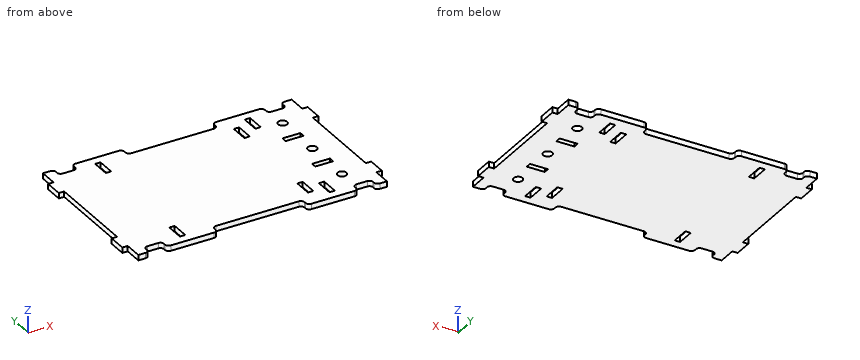
Autodesk Inventor part; units mm, degrees
ref_plane "YZ Plane" through (0, 0, 0) normal (1, 0, 0) x (0, 1, 0)
ref_plane "XZ Plane" through (0, 0, 0) normal (0, 1, 0) x (-1, 0, 0)
ref_plane "XY Plane" through (0, 0, 0) normal (0, 0, 1) x (1, 0, 0)
sketch "Sketch1" plane through (0, 0, 0) normal (0, 0, 1) x (1, 0, 0)
  line L0 (138, 80) -> (141, 80)
  line L1 (141, 80) -> (141, 70)
  line L2 (141, 70) -> (138, 70)
  line L3 (138, 10) -> (141, 10)
  line L4 (141, 10) -> (141, 20)
  line L5 (141, 20) -> (138, 20)
  line L6 (138, 80) -> (138, 90)
  line L7 (138, 20) -> (138, 70)
  line L8 (0, 80) -> (-3, 80)
  line L9 (-3, 80) -> (-3, 70)
  line L10 (-3, 70) -> (0, 70)
  line L11 (0, 20) -> (-3, 20)
  line L12 (-3, 20) -> (-3, 10)
  line L13 (-3, 10) -> (0, 10)
  line L14 (0, 90) -> (0, 80)
  line L15 (0, 70) -> (0, 20)
  line L16 (0, 10) -> (0, 0)
  line L17 (26, 85) -> (29, 85)
  line L18 (29, 85) -> (29, 75)
  line L19 (29, 75) -> (26, 75)
  line L20 (26, 75) -> (26, 85)
  line L21 (26, 15) -> (29, 15)
  line L22 (29, 15) -> (29, 5)
  line L23 (29, 5) -> (26, 5)
  line L24 (26, 5) -> (26, 15)
  line L25 (109, 85) -> (112, 85)
  line L26 (112, 85) -> (112, 75)
  line L27 (112, 75) -> (109, 75)
  line L28 (109, 75) -> (109, 85)
  line L29 (109, 15) -> (112, 15)
  line L30 (112, 15) -> (112, 5)
  line L31 (112, 5) -> (109, 5)
  line L32 (109, 5) -> (109, 15)
  line L33 (16, 88) -> (16, 87)
  line L34 (14, 85) -> (8, 85)
  line L35 (6, 87) -> (6, 88)
  line L36 (94, 88) -> (94, 87)
  line L37 (92, 85) -> (46, 85)
  line L38 (44, 87) -> (44, 88)
  line L39 (132, 88) -> (132, 87)
  line L40 (130, 85) -> (124, 85)
  line L41 (122, 87) -> (122, 88)
  line L42 (138, 90) -> (134, 90)
  line L43 (0, 90) -> (4, 90)
  line L44 (18, 90) -> (42, 90)
  line L45 (96, 90) -> (120, 90)
  line L46 (16, 2) -> (16, 3)
  line L47 (14, 5) -> (8, 5)
  line L48 (6, 3) -> (6, 2)
  line L49 (94, 2) -> (94, 3)
  line L50 (92, 5) -> (46, 5)
  line L51 (44, 3) -> (44, 2)
  line L52 (132, 2) -> (132, 3)
  line L53 (130, 5) -> (124, 5)
  line L54 (122, 3) -> (122, 2)
  line L55 (96, 0) -> (120, 0)
  line L56 (0, 0) -> (4, 0)
  line L57 (18, 0) -> (42, 0)
  arc A0 (4, 0) -> (6, 2) centre (4, 2) ccw
  arc A1 (8, 5) -> (6, 3) centre (8, 3) ccw
  arc A2 (16, 3) -> (14, 5) centre (14, 3) ccw
  arc A3 (16, 2) -> (18, 0) centre (18, 2) ccw
  arc A4 (42, 0) -> (44, 2) centre (42, 2) ccw
  arc A5 (46, 5) -> (44, 3) centre (46, 3) ccw
  arc A6 (94, 3) -> (92, 5) centre (92, 3) ccw
  arc A7 (94, 2) -> (96, 0) centre (96, 2) ccw
  arc A8 (120, 0) -> (122, 2) centre (120, 2) ccw
  arc A9 (124, 5) -> (122, 3) centre (124, 3) ccw
  arc A10 (132, 3) -> (130, 5) centre (130, 3) ccw
  arc A11 (132, 2) -> (134, 0) centre (134, 2) ccw
  arc A12 (6, 88) -> (4, 90) centre (4, 88) ccw
  arc A13 (6, 87) -> (8, 85) centre (8, 87) ccw
  arc A14 (14, 85) -> (16, 87) centre (14, 87) ccw
  arc A15 (18, 90) -> (16, 88) centre (18, 88) ccw
  arc A16 (44, 88) -> (42, 90) centre (42, 88) ccw
  arc A17 (44, 87) -> (46, 85) centre (46, 87) ccw
  arc A18 (92, 85) -> (94, 87) centre (92, 87) ccw
  arc A19 (96, 90) -> (94, 88) centre (96, 88) ccw
  arc A20 (122, 88) -> (120, 90) centre (120, 88) ccw
  arc A21 (122, 87) -> (124, 85) centre (124, 87) ccw
  arc A22 (130, 85) -> (132, 87) centre (130, 87) ccw
  arc A23 (134, 90) -> (132, 88) centre (134, 88) ccw
  line L58 (138, 10) -> (138, 0)
  line L59 (138, 0) -> (134, 0)
  line L60 (103, 10) -> (100, 10)
  line L61 (100, 10) -> (100, 20)
  line L62 (100, 20) -> (103, 20)
  line L63 (103, 20) -> (103, 10)
  line L64 (103, 80) -> (100, 80)
  line L65 (100, 80) -> (100, 70)
  line L66 (100, 70) -> (103, 70)
  line L67 (103, 70) -> (103, 80)
  line L68 (115.5, 60.5) -> (125.5, 60.5)
  line L69 (125.5, 60.5) -> (125.5, 57.5)
  line L70 (125.5, 57.5) -> (115.5, 57.5)
  line L71 (115.5, 57.5) -> (115.5, 60.5)
  line L72 (115.5, 32.5) -> (125.5, 32.5)
  line L73 (125.5, 32.5) -> (125.5, 29.5)
  line L74 (125.5, 29.5) -> (115.5, 29.5)
  line L75 (115.5, 29.5) -> (115.5, 32.5)
  circle A24 centre (123, 45) radius 2.5
  circle A25 centre (123, 73) radius 2.5
  circle A26 centre (123, 17) radius 2.5
  point P0 (16, 85)
  point P1 (6, 85)
  point P2 (94, 85)
  point P3 (44, 85)
  point P4 (132, 85)
  point P5 (122, 85)
  point P6 (16, 5)
  point P7 (6, 5)
  point P8 (94, 5)
  point P9 (44, 5)
  point P10 (132, 5)
  point P11 (122, 5)
  dimension "d1" = 90
  dimension "d3" = 10
  dimension "d4" = 50
  dimension "d5" = 10
  dimension "d10" = 3
  dimension "d11" = 3
  dimension "d13" = 3
  dimension "d14" = 3
  dimension "d16" = 10
  dimension "d17" = 10
  dimension "d20" = 138
  dimension "d21" = 50
  dimension "d22" = 3
  dimension "d23" = 3
  dimension "d24" = 3
  dimension "d27" = 26
  dimension "d28" = 3
  dimension "d30" = 3
  dimension "d31" = 26
  dimension "d33" = 10
  dimension "d34" = 10
  dimension "d35" = 26
  dimension "d36" = 3
  dimension "d38" = 10
  dimension "d39" = 3
  dimension "d40" = 10
  dimension "d45" = 10
  dimension "d46" = 50
  dimension "d47" = 10
  dimension "d48" = 6
  dimension "d49" = 6
  dimension "d54" = 10
  dimension "d55" = 50
  dimension "d56" = 10
  dimension "d57" = 2
  dimension "d58" = 26
  dimension "d59" = 6
  dimension "d60" = 6
  dimension "d62" = 28
  dimension "d63" = 3
  dimension "d64" = 28
  dimension "d65" = 28
  dimension "d66" = 28
  dimension "d67" = 5
  dimension "d68" = 5
  dimension "d69" = 5
  dimension "d70" = 5
  dimension "d71" = 5
  dimension "d72" = 5
  dimension "d73" = 5
  dimension "d74" = 5
  dimension "d75" = 5
  dimension "d76" = 5
  dimension "d77" = 5
  dimension "d78" = 5
  dimension "d79" = 3
  dimension "d80" = 10
  dimension "d81" = 35
  dimension "d82" = 10
  dimension "d83" = 3
  dimension "d84" = 10
  dimension "d85" = 10
  dimension "d86" = 35
  dimension "d89" = 10
extrude "Extrusion5" add sketch "Sketch1" along normal blind 3
properties part number "OpenROV 2.3 Dev EChassis Main Plate"
Can you work these out from the model? Positions are in its coordinate system, mm. Coordinates: 2 decimals unless noted, no trailing zeros. Loops run counter-clockwise (first coordinate to the right, second up) from the corner with the lowest first, then second, coordinate; pieces in that order, holes last.
Item 1: I'm going to push flat-ended pins straight in: pin 1 (0.9 mm diameter, centred on x = -1, z = 2, fed in from +Y); pin 2 (1.5 mm diameter, centred on y = 83.5, z = 2, fed in from +X); pin 3 (1.5 mm diameter, centred on x = 139, z = 1.5, fed in from -Y); pin 4 (4.5 mm diameter, centred on x = 123, y = 17, fed in from +Z). Where does each tip first touch, or does it pass through?
Answers below:
pin 1: stops at y = 80
pin 2: stops at x = 138
pin 3: stops at y = 10
pin 4: passes through
Item 2: Suppose I cut it at B-B (x = 27.5). Please give me the cut outline in (y, z), then the cut area to 3 significant figures.
Answers below:
outline: (0, 0) - (5, 0) - (5, 3) - (0, 3) - close; (15, 0) - (75, 0) - (75, 3) - (15, 3) - close; (85, 0) - (90, 0) - (90, 3) - (85, 3) - close
area: 210 mm2
Item 3: Suppose I cut it at D-D (x = 65.5). Please give me the cut outline in (y, z), then the cut area to 3 significant figures.
Answers below:
outline: (5, 0) - (85, 0) - (85, 3) - (5, 3) - close
area: 240 mm2
Item 4: Please list where these lines run through material, in increasing order: L1, parallel to X at y = 13, z = 1.75; L2, parallel to Y at x = 123, z = 1.05; L3, parallel to X at y = 50, z = 0.5.
Answers below:
L1: x = -3 to 26, 29 to 100, 103 to 109, 112 to 141
L2: y = 4.73 to 14.5, 19.5 to 29.5, 32.5 to 42.5, 47.5 to 57.5, 60.5 to 70.5, 75.5 to 85.27
L3: x = 0 to 138
Item 5: Suppose I cut it at C-C (y = 73). Please give me the cut outline in (x, z).
Answers below:
outline: (-3, 0) - (100, 0) - (100, 3) - (-3, 3) - close; (103, 0) - (120.5, 0) - (120.5, 3) - (103, 3) - close; (125.5, 0) - (141, 0) - (141, 3) - (125.5, 3) - close
Item 6: Suppose I cut it at A-A (y = 45). Please give me the cut outline in (x, z), then the cut area to 3 significant figures.
Answers below:
outline: (0, 0) - (120.5, 0) - (120.5, 3) - (0, 3) - close; (125.5, 0) - (138, 0) - (138, 3) - (125.5, 3) - close
area: 399 mm2
